```python
from build123d import *

# Parameters (mm, degrees)
SKETCH1_R           = 0.61
SKETCH1_R_2         = 0.5
BOSS_EXTRUDE1_DEPTH = 6
SKETCH2_R           = 0.79
BOSS_EXTRUDE2_DEPTH = 2.5
SKETCH3_R           = 0.38
BOSS_EXTRUDE3_DEPTH = 5
FILLET1_R           = 0.35
FILLET2_R           = 0.35


with BuildPart() as part:
    # Sketch1 → Boss-Extrude1 (new body)
    with BuildSketch(Plane(origin=(0, 0, 0), x_dir=(1, 0, 0), z_dir=(0, 1, 0))):
        Circle(SKETCH1_R)
        Circle(SKETCH1_R_2, mode=Mode.SUBTRACT)
    extrude(amount=BOSS_EXTRUDE1_DEPTH)

    # Sketch2 → Boss-Extrude2 (add)
    with BuildSketch(Plane(origin=(0, 6, 0), x_dir=(1, 0, 0), z_dir=(0, 1, 0))):
        Circle(SKETCH2_R)
    extrude(amount=BOSS_EXTRUDE2_DEPTH)

    # Sketch3 → Boss-Extrude3 (add)
    with BuildSketch(Plane(origin=(0, 8.5, 0), x_dir=(1, 0, 0), z_dir=(0, 1, 0))):
        Circle(SKETCH3_R)
    extrude(amount=BOSS_EXTRUDE3_DEPTH)

    # Fillet1
    fillet1_edges = [part.edges().sort_by_distance(p)[0] for p in [
        (-0.38, 13.5, 0),
    ]]
    fillet(fillet1_edges, radius=FILLET1_R)

    # Fillet2
    fillet2_edges = [part.edges().sort_by_distance(p)[0] for p in [
        (-0.38, 8.5, 0),
    ]]
    fillet(fillet2_edges, radius=FILLET2_R)


solid = part.part
```
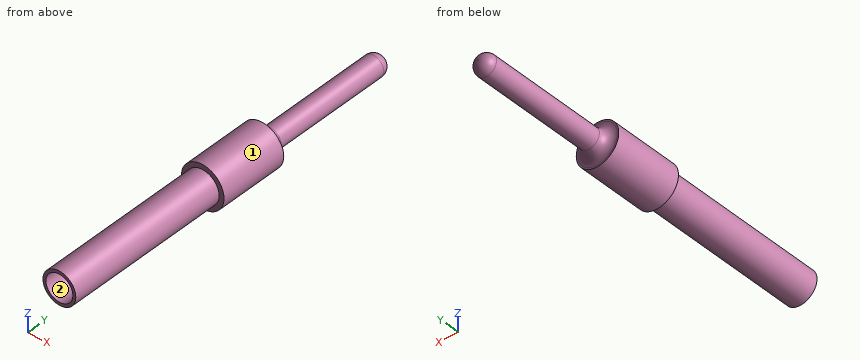
Can you work these out from the model? Positions are in its coordinate system, mm. Face numbers are marked on the shaded views. Round coordinates to 2 decimals unless told otherwise and drop trailing zeros. Loops run counter-clockwise (first coordinate to the right, second up) from the corner with the lowest first, then second, coordinate; pieces in that order, holes last. Notation, with made-up numbers: M 21.25,67 L 48.25,67 A16 cw 48.25,83 Z; hole C -17,-38.5 d10. An arc over 180 degrees is marked long. Answer as a JSON object with one key per item and string values. Group by question number.
Q1. Imagine slicing it at C-C, the plane y = 7.75. Please give me the cut outline in (x, z).
Q2. Imagine slicing it at A-A, the plane y = 3. Please give me the cut outline in (x, z).
Q3. We'd pull the mould along X, two halves only. Please class the marked faces 1 and 2: +X half, -X half, draft (parallel to the pull), parting line (faces both ways), or undercut.
Q4. Please list where these lines run through material, in increasing order: L1, parallel to Y at x = 0.45, z = 0.6; L2, parallel to X at y = 5.25, z = -0.4; L3, parallel to Z at x = -0.2, y = 9.75.
Q5. Imagine slicing it at B-B, the plane y = 10.25. Please give me the cut outline in (x, z), then the cut area to 3 significant figures.
Findings:
{
 "1": {"outline": "C 0,0 d1.58"},
 "2": {"outline": "C 0,0 d1.22; hole C 0,0 d1"},
 "3": {"face 1": "parting line", "face 2": "undercut"},
 "4": {"L1": "y = 6 to 8.5", "L2": "x = -0.46 to -0.3, 0.3 to 0.46", "L3": "z = -0.32 to 0.32"},
 "5": {"outline": "C 0,0 d0.76", "area": "0.454 mm2"}
}
